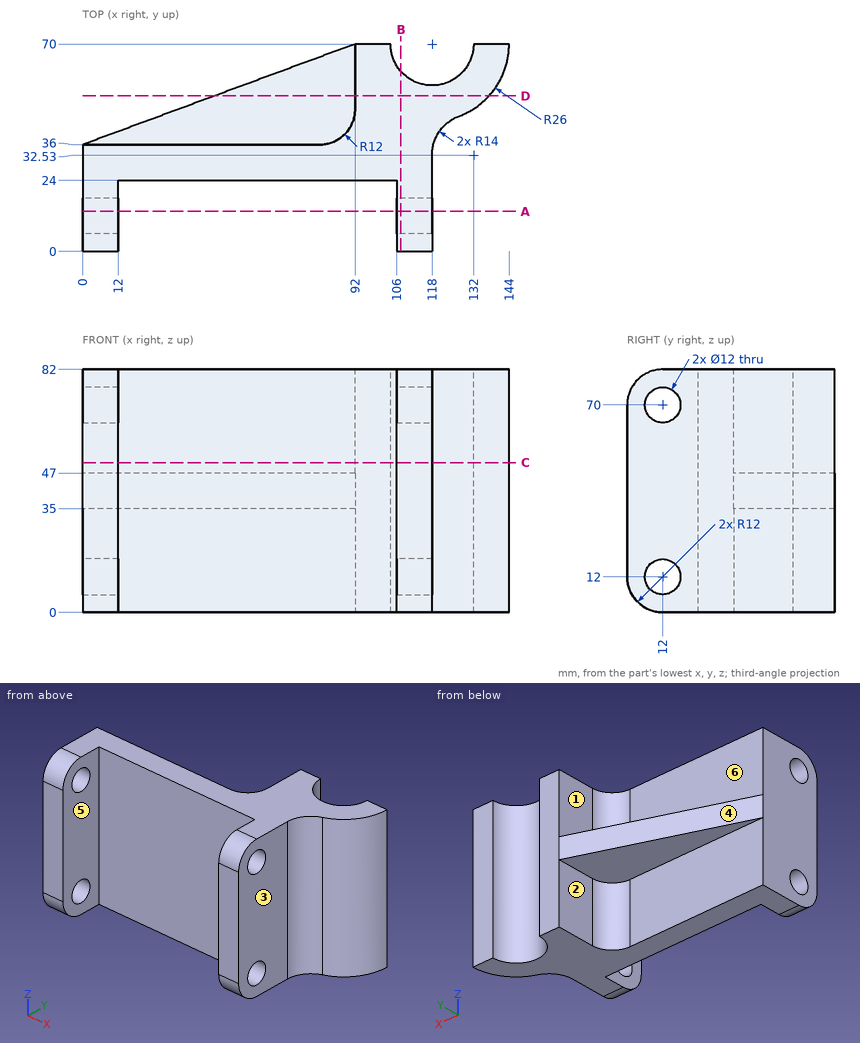
Input: dimensioned drawing with shaded views. Units: mm. Origin: part minimum x, y, z. A direction names the side the tool comes from. Round coordinates to 2 decimals unless told otherwise and drop trailing zeros. Order: outer loops, then holes, each group sorted by start corner. A loop starts at its lowest first (then second) coordinate and runs counter-clockwise, first axis right, second up.
1. Pin query (flat end, axial travel): P1, Ø1.5, axis at x = 109.5, z = 32.5, coming from the +Y side; P2, Ø16.5, axis at y = 12, z = 33, coming from the +X side; P3, Ø5, axis at x = 91.5, z = 63, coming from the -Y side. Return the tip coordinate at first contact, or that it passes through.
The answers:
P1: stops at y = 59.49
P2: stops at x = 118
P3: stops at y = 24
2. Set-up query: the marked faces 1, 2 and 3. Return all of +Z, -Z, +X, -X, +Y, -Y with unobstructed straight access to the full face (end or side cutting, diameter ignored); none if empty.
The answers:
face 1: +Z, -X, +Y
face 2: -Z, -X, +Y
face 3: +Z, -Z, +X, -Y
3. Material intervals for line 1 (Z direction, x = 110.5, y = 12); line 2 (X direction, y = 19.5, z = 72); line 3 (Y direction, x = 8.5, z = 12), sorted ascending.
The answers:
line 1: z = 0 to 6, 18 to 64, 76 to 82
line 2: x = 0 to 12, 106 to 118
line 3: y = 0 to 6, 18 to 36
4. Cut plane A-A, the plane y = 13.5. Output: boundary loops of the cut face in (x, z).
The answers:
outline: (0, 0) - (12, 0) - (12, 6.19) - (0, 6.19) - close; (0, 17.81) - (12, 17.81) - (12, 64.19) - (0, 64.19) - close; (0, 75.81) - (12, 75.81) - (12, 82) - (0, 82) - close; (106, 0) - (118, 0) - (118, 6.19) - (106, 6.19) - close; (106, 17.81) - (118, 17.81) - (118, 64.19) - (106, 64.19) - close; (106, 75.81) - (118, 75.81) - (118, 82) - (106, 82) - close
5. Mould query, pull axis X, two halves, no side actions, for the marked faces 4, 5 and 6. Classes: released by +X, released by -X, zero draft, split by the parting line, or undercut.
The answers:
face 4: released by -X
face 5: undercut
face 6: zero draft
6. Cut plane B-B, the plane x = 107.5. Output: boundary loops of the cut face in (y, z), then the cut area to 3 significant figures.
The answers:
outline: (0, 12) arc R12 ccw to (12, 0) - (60.74, 0) - (60.74, 82) - (12, 82) arc R12 ccw to (0, 70) - close; hole circle Ø12 at (12, 12); hole circle Ø12 at (12, 70)
area: 4,690 mm2
7. Cut plane D-D, the plane y = 52.5. Output: boundary loops of the cut face in (x, z).
The answers:
outline: (44.65, 35) - (92, 35) - (92, 0) - (137.23, 0) - (137.23, 82) - (92, 82) - (92, 47) - (44.65, 47) - close
8. Cut plane C-C, the plane z = 50.5. Output: boundary loops of the cut face in (x, y), then the cut area to 3 significant figures.
The answers:
outline: (0, 0) - (12, 0) - (12, 24) - (106, 24) - (106, 0) - (118, 0) - (118, 32.53) arc R14 cw to (127.1, 45.64) arc R26 ccw to (144, 70) - (132, 70) arc R14 cw to (104, 70) - (92, 70) - (92, 48) arc R12 cw to (80, 36) - (0, 36) - close
area: 3,150 mm2
